Could you check a few things on this model? Use its own coordinates, in mm. Face numbers are marked on the shaded views. A direction names the side the tool comes from. Give positions to 0.01 mm unless a question says otherwise; leave off trailing zeros. Loops run counter-clockwise (first coordinate to the right, second up) from the corner with the lowest first, then second, coordinate; pieces in that order, holes last. Notation, with made-up numbers: (32.5, 37.5) - (38.5, 37.5) arc R25 cw to (38.5, 70.5) - close; hole circle Ø4 at (73.5, 36). An arc over 180 degrees is marked (long way). Write each question's results on one line, items separated by ' | '. Start each with the question number.
1) I'm going to push flat-ended pins straight in: pin 1 (1 mm diameter, centred on x = 18.5, z = 11.5, fed in from -Y); pin 2 (6 mm diameter, centred on x = 7, y = 8, fed in from +Z); pin 3 (2 mm diameter, centred on x = 15.5, y = -15.5, fed in from -Z). Where does each tip first touch, or does it pass through?
2) I want a section at A-A, the plane y = 0. Write out the boundary of the cut face in (x, z).
3) I want a section at B-B, the plane z = 2.25. Write out the boundary of the cut face in (x, y).
4) If I drill on probe 1 along X at (y, z) = (15.5, 3.75); probe 2 along Y at (x, z) = (0, -0.65), over which ranges is the centre line in solid material (lowest first)? Write a range as [from, to].
5) On a 3-axis mill with a long thin cutter (end or side, diameter ignored), from which of +Z, -Z, +X, -X, +Y, -Y can I reach the whole of each face in a straight line? I mean the marked faces 4 and 5. Say none if no direction works.
6) If we mould it in two halves opening along Y, with no side actions, what happens to the marked faces 1, 2 and 3? For each: +Y half, -Y half, draft (parallel to the pull), parting line (faces both ways), or undercut.
7) I want a section at D-D, the plane z = 11.25. Write out the boundary of the cut face in (x, y), and give its area (3 significant figures).
from build123d import *

# Parameters (mm, degrees)
BOSS_EXTRUDE1_DEPTH             = 12.2
SKETCH2_W                       = 2
SKETCH2_H                       = 26
CUT_EXTRUDE1_DEPTH              = 49.516388984
SKETCH3_W                       = 26
SKETCH3_H                       = 2
CUT_EXTRUDE2_DEPTH              = 49.516388984
SKETCH4_R                       = 16.5
CUT_EXTRUDE3_DEPTH              = 0.6
SKETCH5_R                       = 11
BOSS_EXTRUDE2_DEPTH             = 2.6
SKETCH6_R                       = 3.25
CUT_EXTRUDE4_DEPTH              = 2
SKETCH7_R                       = 2.5
CUT_EXTRUDE5_DEPTH              = 33.106697121
FILLET1_R                       = 0.5
FILLET3_R                       = 0.5
FILLET4_R                       = 2
M3X0_5_TAPPED_HOLE1_D           = 2.5
M3X0_5_TAPPED_HOLE1_DEPTH       = 10
M3X0_5_TAPPED_HOLE1_CSINK_D     = 3.5
M3X0_5_TAPPED_HOLE1_CSINK_ANGLE = 90
M3X0_5_TAPPED_HOLE1_TIP         = 0.751075774


with BuildPart() as part:
    # Sketch1 → Boss-Extrude1 (new body)
    with BuildSketch(Plane.XY):
        Polygon((-17.183766184, 21), (-21, 17.183766184), (-21, -17.183766184), (-17.183766184, -21), (17.183766184, -21), (21, -17.183766184), (21, 17.183766184), (17.183766184, 21), align=None)
    extrude(amount=BOSS_EXTRUDE1_DEPTH)

    # Sketch2 → Cut-Extrude1 (cut, through all)
    with BuildSketch(Plane(origin=(21, 0, 0), x_dir=(0, 0, -1), z_dir=(1, 0, 0))):
        with Locations((-11.2, 0)):
            Rectangle(SKETCH2_W, SKETCH2_H)
    extrude(amount=-CUT_EXTRUDE1_DEPTH, mode=Mode.SUBTRACT)

    # Sketch3 → Cut-Extrude2 (cut, through all)
    with BuildSketch(Plane(origin=(0, 21, 0), x_dir=(1, 0, 0), z_dir=(0, 1, 0))):
        with Locations((0, -11.2)):
            Rectangle(SKETCH3_W, SKETCH3_H)
    extrude(amount=-CUT_EXTRUDE2_DEPTH, mode=Mode.SUBTRACT)

    # Sketch4 → Cut-Extrude3 (cut)
    with BuildSketch(Plane(origin=(0, 0, 0), x_dir=(-1, 0, 0), z_dir=(0, 0, -1))):
        Circle(SKETCH4_R)
    extrude(amount=-CUT_EXTRUDE3_DEPTH, mode=Mode.SUBTRACT)

    # Sketch5 → Boss-Extrude2 (add)
    with BuildSketch(Plane(origin=(0, 0, 0.6), x_dir=(-1, 0, 0), z_dir=(0, 0, -1))):
        Circle(SKETCH5_R)
    extrude(amount=BOSS_EXTRUDE2_DEPTH)

    # Sketch6 → Cut-Extrude4 (cut)
    with BuildSketch(Plane(origin=(0, 0, -2), x_dir=(-1, 0, 0), z_dir=(0, 0, -1))):
        Circle(SKETCH6_R)
    extrude(amount=-CUT_EXTRUDE4_DEPTH, mode=Mode.SUBTRACT)

    # Sketch7 → Cut-Extrude5 (cut, through all)
    with BuildSketch(Plane(origin=(0, 0, 0), x_dir=(-1, 0, 0), z_dir=(0, 0, -1))):
        Circle(SKETCH7_R)
    extrude(amount=-CUT_EXTRUDE5_DEPTH, mode=Mode.SUBTRACT)

    # Fillet1
    fillet1_edges = [part.edges().sort_by_distance(p)[0] for p in [
        (3.25, 0, -2),
    ]]
    fillet(fillet1_edges, radius=FILLET1_R)

    # Fillet3
    fillet3_edges = [part.edges().sort_by_distance(p)[0] for p in [
        (11, 0, 0.6),
    ]]
    fillet(fillet3_edges, radius=FILLET3_R)

    # Fillet4
    fillet4_edges = [part.edges().sort_by_distance(p)[0] for p in [
        (17.183766184, 21, 6.1),
        (21, 17.183766184, 6.1),
        (21, -17.183766184, 6.1),
        (17.183766184, -21, 6.1),
        (-17.183766184, -21, 6.1),
        (-21, -17.183766184, 6.1),
        (-21, 17.183766184, 6.1),
        (-17.183766184, 21, 6.1),
    ]]
    fillet(fillet4_edges, radius=FILLET4_R)

    # M3x0.5 Tapped Hole1
    with Locations(Plane(origin=(0, 0, 0), x_dir=(-1, 0, 0), z_dir=(0, 0, -1))):
        with Locations((-15.5, -15.5), (-15.5, 15.5), (15.5, 15.5), (15.5, -15.5)):
            CounterSinkHole(M3X0_5_TAPPED_HOLE1_D / 2, M3X0_5_TAPPED_HOLE1_CSINK_D / 2, depth=M3X0_5_TAPPED_HOLE1_DEPTH, counter_sink_angle=M3X0_5_TAPPED_HOLE1_CSINK_ANGLE)
            with Locations((0, 0, -(M3X0_5_TAPPED_HOLE1_DEPTH + M3X0_5_TAPPED_HOLE1_TIP / 2))):  # 118° drill point
                Cone(0, M3X0_5_TAPPED_HOLE1_D / 2, M3X0_5_TAPPED_HOLE1_TIP, mode=Mode.SUBTRACT)


solid = part.part
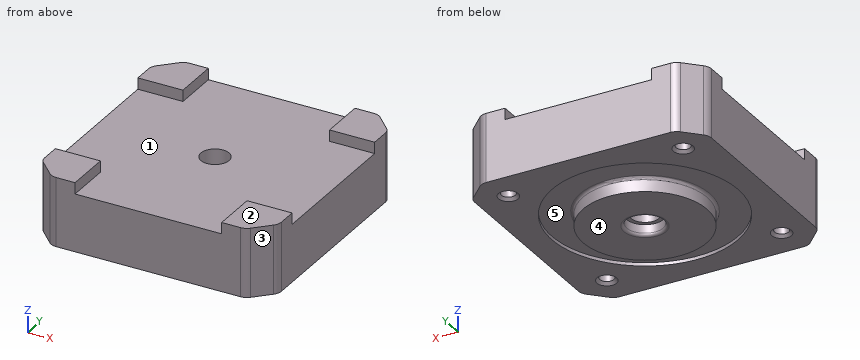
Answers:
1) pin 1: stops at y = -20.18 | pin 2: stops at z = 10.2 | pin 3: stops at z = 10.15
2) outline: (-21, 0) - (-16.5, 0) - (-16.5, 0.6) - (-11.5, 0.6) arc R0.5 cw to (-11, 0.1) - (-11, -2) - (-3.75, -2) arc R0.5 ccw to (-3.25, -1.5) - (-3.25, 0) - (-2.5, 0) - (-2.5, 10.2) - (-21, 10.2) - close; (2.5, 0) - (3.25, 0) - (3.25, -1.5) arc R0.5 ccw to (3.75, -2) - (11, -2) - (11, 0.1) arc R0.5 cw to (11.5, 0.6) - (16.5, 0.6) - (16.5, 0) - (21, 0) - (21, 10.2) - (2.5, 10.2) - close
3) outline: (-21, -16.36) arc R2 ccw to (-20.41, -17.77) - (-17.77, -20.41) arc R2 ccw to (-16.36, -21) - (16.36, -21) arc R2 ccw to (17.77, -20.41) - (20.41, -17.77) arc R2 ccw to (21, -16.36) - (21, 16.36) arc R2 ccw to (20.41, 17.77) - (17.77, 20.41) arc R2 ccw to (16.36, 21) - (-16.36, 21) arc R2 ccw to (-17.77, 20.41) - (-20.41, 17.77) arc R2 ccw to (-21, 16.36) - close; hole circle Ø2.5 at (-15.5, -15.5); hole circle Ø2.5 at (-15.5, 15.5); hole circle Ø5 at (0, 0); hole circle Ø2.5 at (15.5, -15.5); hole circle Ø2.5 at (15.5, 15.5)
4) probe 1: x = [-21, -16.75], [-14.25, 14.25], [16.75, 21] | probe 2: y = [-11, -3.25], [3.25, 11]
5) face 4: -Z, +X, -X, +Y, -Y | face 5: -Z
6) face 1: undercut | face 2: draft | face 3: -Y half
7) outline: (-21, -16.36) arc R2 ccw to (-20.41, -17.77) - (-17.77, -20.41) arc R2 ccw to (-16.36, -21) - (-13, -21) - (-13, -13) - (-21, -13) - close; (-21, 13) - (-13, 13) - (-13, 21) - (-16.36, 21) arc R2 ccw to (-17.77, 20.41) - (-20.41, 17.77) arc R2 ccw to (-21, 16.36) - close; (13, -21) - (16.36, -21) arc R2 ccw to (17.77, -20.41) - (20.41, -17.77) arc R2 ccw to (21, -16.36) - (21, -13) - (13, -13) - close; (13, 13) - (21, 13) - (21, 16.36) arc R2 ccw to (20.41, 17.77) - (17.77, 20.41) arc R2 ccw to (16.36, 21) - (13, 21) - close | area: 226 mm2
